CAD build for the part. Positions are in the model's coordinates, mm. A direction names the side the tool comes from. Round coordinates to 2 decimals unless told otherwise and drop trailing zeros. Loops run counter-clockwise (first coordinate to the right, second up) from the corner with the lowest first, then second, coordinate; pieces in that order, holes last. Notation, with made-up numbers: (15.5, -13) - (64.5, -13) arc R27 ccw to (64.5, 16) - close; hole circle Ø10 at (41, -28.5). An arc over 180 degrees is marked (long way). One line per question, with ' | ' between items.
Autodesk Inventor part; units mm, degrees
ref_plane "YZ Plane" through (0, 0, 0) normal (1, 0, 0) x (0, 1, 0)
ref_plane "XZ Plane" through (0, 0, 0) normal (0, 1, 0) x (-1, 0, 0)
ref_plane "XY Plane" through (0, 0, 0) normal (0, 0, 1) x (1, 0, 0)
sketch "Sketch1" plane through (0, 0, 0) normal (0, 0, 1) x (1, 0, 0)
  line L0 (93.3916, -12.6) -> (93.3916, 12.6)
  line L1 (53.9763, -12.6) -> (93.3916, -12.6)
  line L2 (53.9763, -15.2) -> (53.9763, -12.6)
  line L3 (38.2753, -15.2) -> (53.9763, -15.2)
  line L4 (38.2753, -15.2) -> (23.4296, -15.2)
  line L5 (23.4296, -12.6) -> (23.4296, -15.2)
  line L6 (-76.0546, -12.6) -> (23.4296, -12.6)
  line L7 (23.4296, 12.6) -> (-76.0546, 12.6)
  line L8 (23.4296, 15.2) -> (23.4296, 12.6)
  line L9 (-76.0546, 12.6) -> (-76.0546, -12.6)
  line L10 (-70.1, 10) -> (-66.9, 10)
  line L11 (-66.9, -10) -> (-70.1, -10)
  line L12 (23.4296, 15.2) -> (53.9763, 15.2)
  line L13 (53.9763, 15.2) -> (53.9763, 12.6)
  line L14 (53.9763, 12.6) -> (93.3916, 12.6)
  line L15 (-77.0546, 13.6) -> (22.4296, 13.6)
  line L16 (22.4296, 13.6) -> (22.4296, 16.2)
  line L17 (22.4296, 16.2) -> (54.9763, 16.2)
  line L18 (54.9763, 16.2) -> (54.9763, 13.6)
  line L19 (54.9763, 13.6) -> (94.3916, 13.6)
  line L20 (94.3916, 13.6) -> (94.3916, -13.6)
  line L21 (94.3916, -13.6) -> (54.9763, -13.6)
  line L22 (54.9763, -13.6) -> (54.9763, -16.2)
  line L23 (54.9763, -16.2) -> (38.2753, -16.2)
  line L24 (38.2753, -16.2) -> (22.4296, -16.2)
  line L25 (22.4296, -16.2) -> (22.4296, -13.6)
  line L26 (22.4296, -13.6) -> (-77.0546, -13.6)
  line L27 (-77.0546, -13.6) -> (-77.0546, 13.6)
  line L28 (22.4296, -16.2) -> (22.4296, -20.2) construction
  line L29 (22.4296, -20.2) -> (-87.5704, -20.2)
  line L30 (-87.5704, -20.2) -> (-87.5704, 20.2)
  line L31 (-87.5704, 20.2) -> (22.4296, 20.2)
  line L32 (104.4296, -20.2) -> (22.4296, -20.2)
  line L33 (22.4296, 20.2) -> (104.4296, 20.2)
  line L34 (104.4296, 20.2) -> (104.4296, -20.2)
  circle A0 centre (-82.5704, 17.2) radius 1.6
  circle A1 centre (-82.5704, -17.2) radius 1.6
  circle A2 centre (99.4296, 17.2) radius 1.6
  circle A3 centre (99.4296, -17.2) radius 1.6
  dimension "d0" = 1
  dimension "d1" = 4
  dimension "d2" = 110
  dimension "d3" = 40.4
  dimension "d5" = 82
  dimension "d18" = 5
  dimension "d19" = 5
  dimension "d20" = 3
  dimension "d21" = 3
  dimension "d22" = 5
  dimension "d23" = 3
  dimension "d24" = 5
  dimension "d25" = 3
extrude "Extrusion1" add sketch "Sketch1" against normal blind 4 contours L29 L30 L31 L33 L34 L32
sketch "Sketch2" plane through (0, 0, 0) normal (0, 0, 1) x (1, 0, 0)
  line L0 (79.9, -10) -> (83.1, -10) construction
  line L1 (83.1, 10) -> (79.9, 10) construction
  line L2 (-66.9, -10) -> (-70.1, -10) construction
  line L3 (-70.1, 10) -> (-66.9, 10) construction
  line L4 (81.5, -10) -> (81.5, -13.6) construction
  line L5 (94.3916, -13.6) -> (54.9763, -13.6)
  line L6 (81.5, 10) -> (81.5, 13.6) construction
  line L7 (54.9763, 13.6) -> (94.3916, 13.6)
  line L8 (-68.5, -10) -> (-68.5, -13.6) construction
  line L9 (22.4296, -13.6) -> (-77.0546, -13.6)
  line L10 (-68.5, 10) -> (-68.5, 13.6) construction
  line L11 (-77.0546, 13.6) -> (22.4296, 13.6)
  line L12 (84.25, -10.6) -> (78.75, -10.6)
  line L13 (78.75, -10.6) -> (78.75, -16.6)
  line L14 (78.75, -16.6) -> (84.25, -16.6)
  line L15 (84.25, -16.6) -> (84.25, -10.6)
  line L16 (84.25, -10.6) -> (78.75, -16.6) construction
  line L17 (78.75, -10.6) -> (84.25, -16.6) construction
  line L18 (84.25, 10.6) -> (78.75, 10.6)
  line L19 (78.75, 10.6) -> (78.75, 16.6)
  line L20 (78.75, 16.6) -> (84.25, 16.6)
  line L21 (84.25, 16.6) -> (84.25, 10.6)
  line L22 (84.25, 10.6) -> (78.75, 16.6) construction
  line L23 (78.75, 10.6) -> (84.25, 16.6) construction
  line L24 (-65.75, 10.6) -> (-71.25, 10.6)
  line L25 (-71.25, 10.6) -> (-71.25, 16.6)
  line L26 (-71.25, 16.6) -> (-65.75, 16.6)
  line L27 (-65.75, 16.6) -> (-65.75, 10.6)
  line L28 (-65.75, 10.6) -> (-71.25, 16.6) construction
  line L29 (-71.25, 10.6) -> (-65.75, 16.6) construction
  line L30 (-65.75, -10.6) -> (-71.25, -10.6)
  line L31 (-71.25, -10.6) -> (-71.25, -16.6)
  line L32 (-71.25, -16.6) -> (-65.75, -16.6)
  line L33 (-65.75, -16.6) -> (-65.75, -10.6)
  line L34 (-65.75, -10.6) -> (-71.25, -16.6) construction
  line L35 (-71.25, -10.6) -> (-65.75, -16.6) construction
  point P0 (0, 0)
  point P1 (-71.25, 13.6)
  point P2 (-65.75, 13.6)
  point P3 (-65.75, -13.6)
  point P4 (-71.25, -13.6)
  point P5 (78.75, 13.6)
  point P6 (84.25, 13.6)
  point P7 (84.25, -13.6)
  point P8 (78.75, -13.6)
  dimension "d8" = 5.5
  dimension "d9" = 6
  dimension "d10" = 5.5
  dimension "d11" = 6
  dimension "d12" = 5.5
  dimension "d13" = 6
  dimension "d14" = 5.5
  dimension "d15" = 6
extrude "Extrusion2" cut sketch "Sketch2" against normal blind 4 contours L15 L14 L13 L5 | L19 L20 L21 L7 | L33 L32 L31 L9 | L25 L26 L27 L11
sketch "Sketch4" plane through (-71.25, 16.6, 0) normal (0, -1, 0) x (1, 0, 0)
  line L0 (0, 0) -> (0, -4) construction
  line L1 (5.5, -4) -> (0, -4) construction
  line L2 (150, -4) -> (5.5, -4) construction
  line L3 (155.5, -4) -> (150, -4) construction
  line L4 (169.1963, -4) -> (155.5, -4) construction
  line L5 (169.1963, 0) -> (169.1963, -4) construction
  line L6 (155.5, 0) -> (169.1963, 0) construction
  line L7 (155.5, -4) -> (155.5, 0) construction
  line L8 (0, 0) -> (5.5, 0) construction
  line L9 (-9.8372, 0) -> (0, 0) construction
  line L10 (-9.8372, -4) -> (-9.8372, 0) construction
  line L11 (0, -4) -> (-9.8372, -4) construction
  line L12 (5.5, -4) -> (5.5, 0) construction
  line L13 (150, 0) -> (150, -4) construction
  line L14 (5.5, 0) -> (150, 0) construction
  line L15 (150, 0) -> (155.5, 0) construction
  line L16 (175.6796, -4) -> (172.1628, -4) construction
  line L17 (172.1628, -4) -> (172.1628, 0) construction
  line L18 (172.1628, 0) -> (175.6796, 0) construction
  line L19 (175.6796, 0) -> (175.6796, -4) construction
  line L20 (-12.8037, -4) -> (-16.3204, -4)
  line L21 (-16.3204, -4) -> (-16.3204, 0)
  line L22 (-16.3204, 0) -> (-12.8037, 0)
  line L23 (-12.8037, 0) -> (-12.8037, -4)
  line L24 (0, 0) -> (5.5, 0) construction
  line L25 (2.75, 0) -> (2.75, -2.75) construction
  line L26 (150, 0) -> (155.5, 0) construction
  line L27 (152.75, 0) -> (152.75, -2.75) construction
  point P0 (71.25, 0)
  dimension "d26" = 2.75
  dimension "d27" = 2.75
properties part number "Template-Fixture-Mid" material "Polycarbonate, Clear"
(1) Tool access for faces 1 (the face through (89, -13.6, -2)), 2 (the face through (-14, 14, -4)): list every direction of +Z, -Z, +X, -X, +Y, -Y with a clear straight run to the whole face (end or side of a thin tool).
Results found:
face 1: +Z, -Z | face 2: -Z, +X, -X, +Y, -Y
(2) Cut at C-C, the plane z = -1.2. State how many separate pieces and enclosed holes the cut face has, then the cut area to 3 significant figures.
Results found:
separate pieces: 1 | enclosed holes: 5 | area: 2,830 mm²
(3) Probe L1, parallel to X at y = 15, z = -3.05; L2, parallel to Y at x = 6.5, z = -0.6; L3, parallel to X at y = -6, z = -2.45. List the from-to ranges inside material, lowest first.
Results found:
L1: x = -87.57 to -71.25, -65.75 to 22.43, 54.98 to 78.75, 84.25 to 104.43 | L2: y = -20.2 to -13.6, 13.6 to 20.2 | L3: x = -87.57 to -77.05, 94.39 to 104.43
(4) Two-plate mould, pull along Y, no slides. Class faces 3 (the face through (84.25, 15, -2)), 4 (the face through (-14, 14, 0)), 5 (the face through (10, -20.2, -2)): released by +Y, released by -Y, zero draft, split by the parting line, or undercut.
Results found:
face 3: undercut | face 4: zero draft | face 5: released by -Y
(5) Cut at A-A, the plane x = 39. Write the cut outline in (y, z).
Results found:
outline: (-20.2, -4) - (-16.2, -4) - (-16.2, 0) - (-20.2, 0) - close; (16.2, -4) - (20.2, -4) - (20.2, 0) - (16.2, 0) - close
(6) Cut at B-B, the plane y = -12. Write the cut outline in (x, z).
Results found:
outline: (-87.57, -4) - (-77.05, -4) - (-77.05, 0) - (-87.57, 0) - close; (94.39, -4) - (104.43, -4) - (104.43, 0) - (94.39, 0) - close
